The drawing under review shows one solid part. Ordinate dimensions are in mm from its lowest x, y, z. A direction names the side the tool comes from. Give positions to 0.01 mm unless a question says otherwise; leave off trailing zeros. Loops run counter-clockwise (first coordinate to the right, second up) from the corner with the lowest first, then second, coordinate; pieces in that order, holes last. Notation, with made-up numbers: M 50.25,-8.75 L 74.25,-8.75 A23 cw 74.25,13.25 Z; hole C -8.75,0.25 d1. An arc over 180 degrees is marked long. Put each result on its own line as item: value. Start each with the question number.
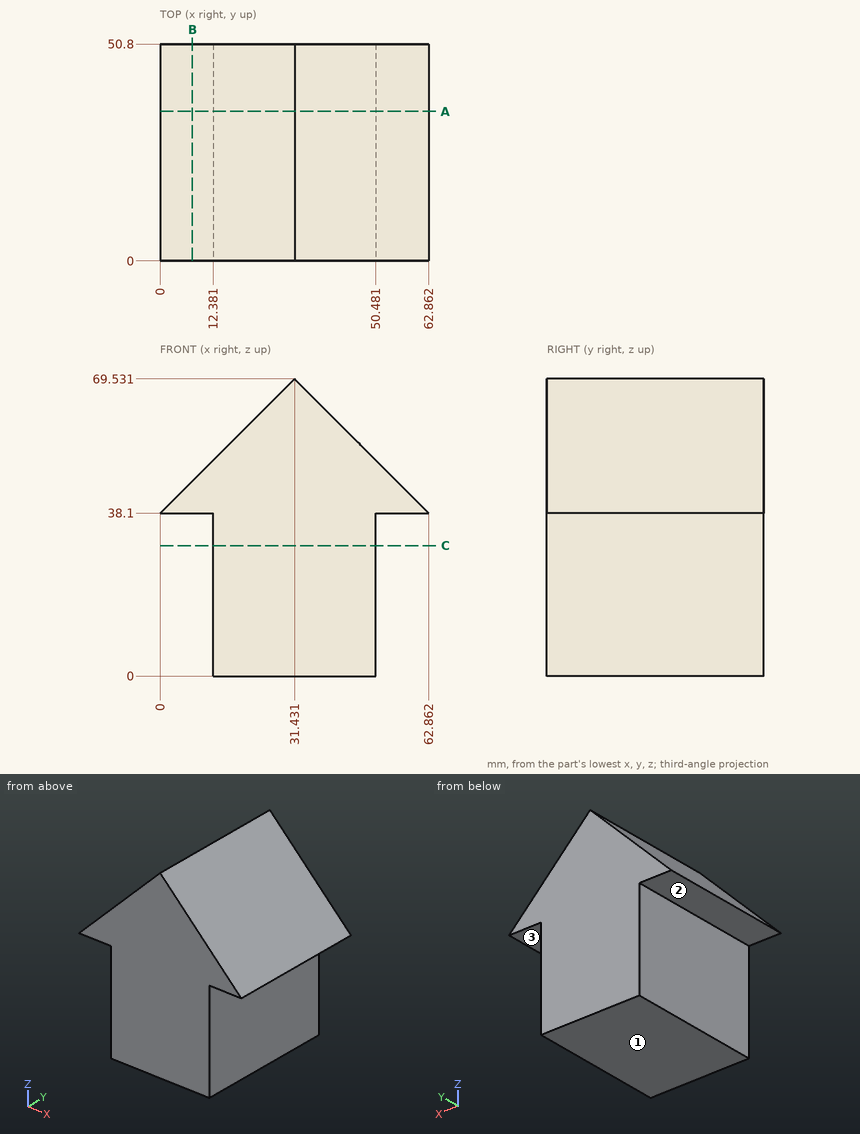
(1) For the marked faces 1, 2 and 3, list the 3-axis set-ups (+Z, -Z, +X, -X, +Y, -Y) from which the entire face can be reached by the end or side of a thin tool; tool diameter is ignored.
(2) We need section C-C, the plane z = 30.5. Write out the cut boundary in (x, y), plus the area to 3 significant figures.
(3) To check wall thickness, follow L1, parallel to X at y = 44, z = 17.5; L2, parallel to Z at x = 18.5, y = 27.5; L3, parallel to Z at x = 38.5, y = 19. State the ranges of each line that lie inside material, in increasing order. Write a range as [from, to].
(4) We need section B-B, the plane x = 7.5. Write out the cut boundary in (y, z), plus the area to 3 significant figures.
(5) Insertion check: pin 1 (5 mm diameter, centred on x = 10, y = 25.5, fed in from +Z); pin 2 (8 mm diameter, centred on x = 56.5, y = 32.5, fed in from +Z); pin 3 (19 mm diameter, centred on y = 34, z = 23, fed in from +X). Each pin has a flat end and moves straight along its axis. Give the tip position at first contact, or say it passes through.
(6) We need section A-A, the plane y = 35. Write out the cut boundary in (x, z).
Check sheet entries:
1. face 1: -Z, +X, -X, +Y, -Y
1. face 2: -Z, -X, +Y, -Y
1. face 3: -Z, +X, +Y, -Y
2. outline: M 12.38,0 L 50.48,0 L 50.48,50.8 L 12.38,50.8 Z
2. area: 1,940 mm²
3. L1: x = [12.38, 50.48]
3. L2: z = [0, 56.6]
3. L3: z = [0, 62.46]
4. outline: M 0,38.1 L 50.8,38.1 L 50.8,45.6 L 0,45.6 Z
4. area: 381 mm²
5. pin 1: stops at z = 50.6
5. pin 2: stops at z = 48.46
5. pin 3: stops at x = 50.48
6. outline: M 0,38.1 L 12.38,38.1 L 12.38,0 L 50.48,0 L 50.48,38.1 L 62.86,38.1 L 31.43,69.53 Z
